from build123d import *

# Parameters (mm, degrees)
F0_W     = 24.65
F0_H     = 6
F1_DEPTH = 12.8
F2_W     = 17.15
F2_H     = 5.8
F3_DEPTH = 25
F6_DEPTH = 10.3
F4_R     = 1.3
F7_DEPTH = 25
F8_R     = 1.5
F9_DEPTH = 25


with BuildPart() as f1:
    # F0 (on Top) → F1 (new body)
    with BuildSketch(Plane.XY):
        with Locations((-12.325, 0)):
            Rectangle(F0_W, F0_H)
    extrude(amount=F1_DEPTH)

    # F2 (on face) → F3 (cut)
    with BuildSketch(Plane.XZ.offset(3)):
        with Locations((-8.575, 9.9)):
            Rectangle(F2_W, F2_H)
    extrude(amount=-F3_DEPTH, mode=Mode.SUBTRACT)

    # F5 (on face) → F6 (cut)
    with BuildSketch(Plane(origin=(0, 0, 0), x_dir=(1, 0, 0), z_dir=(0, 0, -1))):
        with BuildLine():
            Line((-24.65, -3), (-22.15, -3))
            ThreePointArc((-22.15, -3), (-19.15, 0), (-22.15, 3))
            Line((-22.15, 3), (-24.65, 3))
            Line((-24.65, 3), (-24.65, -3))
        make_face()
    extrude(amount=-F6_DEPTH, mode=Mode.SUBTRACT)

    # F4 (on face) → F7 (cut)
    with BuildSketch(Plane.XY.offset(12.8)):
        with Locations((-21.65, 0)):
            Circle(F4_R)
    extrude(amount=-F7_DEPTH, mode=Mode.SUBTRACT)

    # F8 (on face) → F9 (cut)
    with BuildSketch(Plane.XZ.offset(3)):
        with Locations((-5, 2.5)):
            Circle(F8_R)
    extrude(amount=-F9_DEPTH, mode=Mode.SUBTRACT)

    # F10: F1 across face


with BuildPart() as f1_1:
    add(f1.part)
    add(f1.part.mirror(Plane(origin=(0, 0, 3.5), x_dir=(0, 1, 0), z_dir=(1, 0, 0))))


solid = f1_1.part
Check sheet for the modelled part. Datum: model origin and axes. Units: mm. A direction names the side the tool comes from. Give positions to 0.01 mm unless a question says otherwise; leave off trailing zeros. Loops run counter-clockwise (first coordinate to the right, second up) from the corner with the lowest first, then second, coordinate; pieces in that order, holes last. Notation, with made-up numbers: M -16.75,31.25 L 10.25,31.25 A26 ccw 10.25,48.25 Z; hole C -7,19.25 d3. An arc over 180 degrees is marked long. Use a Markdown table: item, result. Add a question column.
Q1. Scan lines: line 1 along X through (y, z) = (1.75, 10.5); line 2 along Z through (x, y) = (5, 1.05); line 3 along X through (y, z) = (2.6, 3). Record each from-to range of solid material in increasing order. Write a range as [from, to].
Q2. Sectioned sample at A-A, the plane z = 12. Record the cut outline in (x, y).
Q3. Mould release check, pull along X, two halves, no side actions. Record for faces 1 (the flat face through (24.65, 0, 12)), 2 (the flat face through (17.15, 0, 10)), 3 (the cylindrical face through (6.2, 0, 1.6)), 4 (the flat face through (-23.2, 0, 10.3)): pulls with the +X half, pulls with the -X half, needs draft (parallel to the pull), parting line crosses it, or undercut.
Q4. Go/stop test with flat-tipped pins: pin 1 (3.5 mm diameter, centred on x = 21.65, y = 0, fed in from -Z); pin 2 (1 mm diameter, centred on x = -6.5, y = 2, fed in from +Z). Record where each tip stops, or that it passes through.
Q5. Tool access check on faces 5 (the flat face through (0, 0, 7)), 6 (the cylindrical face through (-19.15, 0.07, 5.08)), 7 (the flat face through (23.2, 0, 10.3)), 8 (the flat face through (-5, 3, 5)). Record the directions out of +Z, -Z, +X, -X, +Y, -Y that give a thin tool (end or side, any length) a straight path to the whole face; none if there is none.
Q6. Sectioned sample at C-C, the plane x = -5. Record the cut outline in (y, z).
Q7. Sectioned sample at B-B, the plane y = 0. Record the cut outline in (x, z).
Q8. Sectioned sample at D-D, the plane y = 2.3. Record the cut outline in (x, z).
Verdict:
| question | item | result |
|---|---|---|
| 1 | line 1 | [-24.65, -17.15], [17.15, 24.65] |
| 1 | line 2 | [0, 1], [4, 7] |
| 1 | line 3 | [-20.65, -6.41], [-3.59, 3.59], [6.41, 20.65] |
| 2 | outline | M -24.65,-3 L -17.15,-3 L -17.15,3 L -24.65,3 Z; M 17.15,-3 L 24.65,-3 L 24.65,3 L 17.15,3 Z; hole C -21.65,0 d2.6; hole C 21.65,0 d2.6 |
| 3 | face 1 | pulls with the +X half |
| 3 | face 2 | undercut |
| 3 | face 3 | undercut |
| 3 | face 4 | needs draft |
| 4 | pin 1 | z = 10.3 |
| 4 | pin 2 | z = 7 |
| 5 | face 5 | +Z, +Y, -Y |
| 5 | face 6 | -Z, -X |
| 5 | face 7 | -Z, +X |
| 5 | face 8 | +Z, -Z, +X, -X, +Y |
| 6 | outline | M -3,0 L 3,0 L 3,1 L -3,1 Z; M -3,4 L 3,4 L 3,7 L -3,7 Z |
| 7 | outline | M -24.65,10.3 L -22.95,10.3 L -22.95,12.8 L -24.65,12.8 Z; M -20.35,10.3 L -19.15,10.3 L -19.15,0 L 19.15,0 L 19.15,10.3 L 20.35,10.3 L 20.35,12.8 L 17.15,12.8 L 17.15,7 L -17.15,7 L -17.15,12.8 L -20.35,12.8 Z; M 22.95,10.3 L 24.65,10.3 L 24.65,12.8 L 22.95,12.8 Z; hole C -5,2.5 d3; hole C 5,2.5 d3 |
| 8 | outline | M -24.65,10.3 L -20.22,10.3 L -20.22,0 L 20.22,0 L 20.22,10.3 L 24.65,10.3 L 24.65,12.8 L 17.15,12.8 L 17.15,7 L -17.15,7 L -17.15,12.8 L -24.65,12.8 Z; hole C -5,2.5 d3; hole C 5,2.5 d3 |
